For this review, take the finished solid that the model builds, in its own axes (mm). A direction names the side the tool comes from. Round coordinates to 2 decimals unless told otherwise and drop trailing zeros. Order: outer loops, then holes, each group sorted by start corner. A loop starts at its lowest first (then second) coordinate and runs counter-clockwise, first axis right, second up. Notation, with made-up numbers: M 13,-9 L 68,-9 A6 ccw 68,-4 Z; hole C 61.25,51.5 d9. An arc over 180 degrees is marked long. Answer as a JSON object with one key per item and string values.
Autodesk Inventor part; units mm, degrees
ref_plane "YZ Plane" through (0, 0, 0) normal (1, 0, 0) x (0, 1, 0)
ref_plane "XZ Plane" through (0, 0, 0) normal (0, 1, 0) x (-1, 0, 0)
ref_plane "XY Plane" through (0, 0, 0) normal (0, 0, 1) x (1, 0, 0)
sketch "Sketch1" plane through (0, 0, 0) normal (0, 1, 0) x (-1, 0, 0)
  line L0 (0, 0) -> (101.6, 0)
  line L1 (101.6, 0) -> (101.6, -101.6)
  line L2 (0, 0) -> (101.6, -101.6)
  dimension "d2" = 101.6
  dimension "d3" = 101.6
extrude "Extrusion1" add sketch "Sketch1" along normal blind 38.1
sketch "Sketch2" plane through (0, 38.1, 0) normal (0, 1, 0) x (1, 0, 0)
  line L0 (-101.6, 0) -> (0, 0)
  line L1 (-101.6, 101.6) -> (-101.6, 0)
  line L2 (-6.35, 6.35) -> (-95.25, 6.35)
  line L3 (-95.25, 6.35) -> (-95.25, 95.25)
  line L4 (0, 0) -> (-101.6, 101.6)
  line L5 (-6.35, 6.35) -> (-95.25, 95.25)
  dimension "d6" = 6.35
extrude "Extrusion2" cut sketch "Sketch2" against normal blind 19.05 contours L2 L3 L4
hole "Hole1" at (-95.25, 28.575, -76.2) direction (-1, 0, 0) diameter 6.35 end through all
hole "Hole2" at (-95.25, 28.575, -25.4) direction (-1, 0, 0) diameter 6.35 end through all
hole "Hole3" at (-25.4, 28.575, -6.35) direction (0, 0, 1) diameter 6.35 end through all
hole "Hole4" at (-76.2, 28.575, -6.35) direction (0, 0, 1) diameter 6.35 end through all
sketch "Sketch3" plane through (0, 0, 0) normal (0, -1, 0) x (1, 0, 0)
  line L0 (-74.5236, -579.4502) -> (246.1514, -579.4502)
  line L1 (-74.5236, -34.9377) -> (-74.5236, -579.4502)
  line L2 (246.1514, -34.9377) -> (-74.5236, -34.9377)
  line L3 (246.1514, -579.4502) -> (246.1514, -34.9377)
  line L4 (-74.5236, -34.9377) -> (-74.5236, -74.5236)
  line L5 (-101.6, -101.6) -> (0, 0)
  line L6 (-34.8701, -34.9377) -> (-74.5236, -34.9377)
  line L7 (-34.8701, -34.9377) -> (-74.5236, -74.5236)
extrude "Extrusion3" cut sketch "Sketch3" against normal blind 9.7282 contours L1 L2 L5 | L5 L2 L7
properties part number "bracket"
1) Insertion check: P1, Ø2, axis at x = -69.5, y = 32.5, coming from the -Z side; P2, Ø6, axis at x = -82.5, y = 10, coming from the -Z side; P3, Ø10, axis at y = 18.5, z = -30, coming from the +X side. Each pin has a flat end and moves straight along its axis. Give the tip position at first contact, or say it passes through.
Geometry check:
{"P1": "stops at z = -6.35", "P2": "stops at z = -85.5", "P3": "stops at x = -25"}
2) Add section B-B on x = -76.2. State the section outline as (y, z) points.
Geometry check:
{"outline": "M 0,-76.2 L 19.05,-76.2 L 19.05,-6.35 L 25.4,-6.35 L 25.4,0 L 0,0 Z; M 31.75,-6.35 L 38.1,-6.35 L 38.1,0 L 31.75,0 Z"}
3) For L1, parallel to Z at x = -46, y = 9; L2, parallel to X at y = 20.5, z = -45; L3, parallel to Y at x = -80, z = -67, list the stretches that pass through material, from the lowest coordinate up.
Geometry check:
{"L1": "z = -34.94 to 0", "L2": "x = -101.6 to -95.25", "L3": "y = 0 to 19.05"}
4) Machinability: for faces 5 (the flat face through (-54, 5, -34.938)), 6 (the flat face through (-73, 38.1, -5)), 7 (the flat face through (-50, 29, -6.35)), which of the approach directions +Z, -Z, +X, -X, +Y, -Y give a long, thin tool a straight path to every point of the face, cutting with its end or side? Answer none if there is none.
Geometry check:
{"face 5": "-Z, +X, -Y", "face 6": "+Z, -Z, +X, -X, +Y", "face 7": "-Z, +X, +Y"}
5) Add section A-A on z = -76.2. State the section outline as (x, y) points.
Geometry check:
{"outline": "M -101.6,0 L -76.2,0 L -76.2,19.05 L -95.25,19.05 L -95.25,25.4 L -101.6,25.4 Z; M -101.6,31.75 L -95.25,31.75 L -95.25,38.1 L -101.6,38.1 Z"}
6) Mouldability with a two-part tool opening along X and no side actions: class faces 1 (the cylindrical face through (-27.546, 26.235, -3.131)), 2 (the flat face through (-59, 9.728, -50)), 3 (the flat face through (-50, 15, -50)), 4 (the cylindrical face through (-78.346, 26.235, -3.131)) as +X half, -X half, draft (parallel to the pull), parting line (faces both ways), or undercut.
Geometry check:
{"face 1": "undercut", "face 2": "draft", "face 3": "+X half", "face 4": "undercut"}
7) Add section C-C on y = 27. State the section outline as (x, z) points, and give its area (3 significant figures).
Geometry check:
{"outline": "M -101.6,-101.6 L -95.25,-95.25 L -95.25,-78.96 L -101.6,-78.96 Z; M -101.6,-73.44 L -95.25,-73.44 L -95.25,-28.16 L -101.6,-28.16 Z; M -101.6,-22.64 L -95.25,-22.64 L -95.25,-6.35 L -78.96,-6.35 L -78.96,0 L -101.6,0 Z; M -73.44,-6.35 L -28.16,-6.35 L -28.16,0 L -73.44,0 Z; M -22.64,-6.35 L -6.35,-6.35 L 0,0 L -22.64,0 Z", "area": "1,070 mm²"}
8) Add section D-D on z = -60. State the section outline as (x, y) points, and give its area (3 significant figures).
Geometry check:
{"outline": "M -101.6,0 L -74.52,0 L -74.52,9.73 L -60,9.73 L -60,19.05 L -95.25,19.05 L -95.25,38.1 L -101.6,38.1 Z", "area": "772 mm²"}
